For this review, take the finished solid that the model builds, in its own axes (mm). Coordinates: 2 decimals unless noted, no trailing zeros. Order: outer loops, then holes, each group sorted by start corner. A loop starts at its lowest first (then second) coordinate and runs counter-clockwise, first axis right, second up. Notation, with made-up numbers: (83.25, 11.25) -> (142.25, 11.25) arc R14 cw to (142.25, 15.25) -> close; hole circle Ø7 at (7.5, -12.75). An arc over 180 degrees is marked (long way). Return JSON: item names as keys, results as strings. Group by question number.
Item 1: Take a section at A-A (x = -3.5). Write out the cut boundary in (y, z), then the cut area to 3 significant figures.
Item 2: Take a section at C-C (y = -8.5). Write out the cut boundary in (x, z).
Item 3: Insertion check: pin 1 (4 mm diameter, centred on x = 14, y = -42, fed in from +Z); pin 2 (8 mm diameter, centred on x = -20.5, z = 17.5, fed in from +Y). Each pin has a flat end and moves straight along its axis. Give the tip position at first contact, or say it passes through.
Item 4: For line 1 along Z through (x, y) = (12, -12); line 2 along Y through (x, z) = (23, 8); line 3 along Y through (x, z) = (26, 11), list the stretches that pass through material, from the lowest coordinate up.
Item 5: Take a section at B-B (z = 20). Write out the cut boundary in (x, y), then the cut area to 3 significant figures.
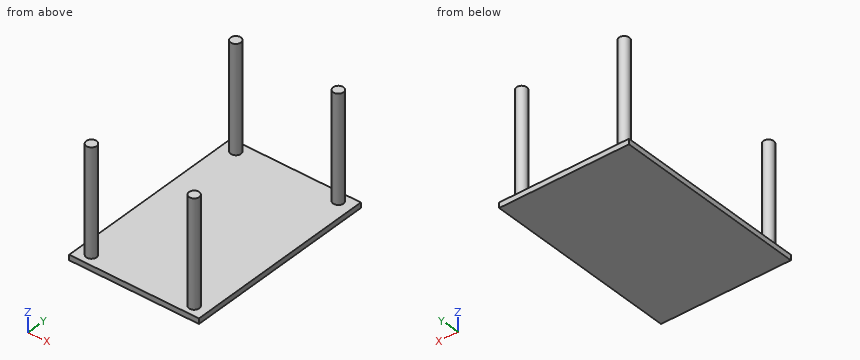
```python
from build123d import *

# Parameters (mm, degrees)
F0_W      = 61.878236
F0_H      = 93.249064
F1_DEPTH  = 2.54
F2_R      = 3.356363
F3_DEPTH  = 34.29
F4_R      = 2.475799
F5_DEPTH  = 50.8
F6_R      = 2.475799
F7_DEPTH  = 50.8
F8_R      = 2.475798
F9_DEPTH  = 50.8
F10_R     = 2.459012
F11_DEPTH = 50.8


with BuildPart() as f1:
    # F0 (on Top) → F1 (new body)
    with BuildSketch(Plane.XY):
        with Locations((-1e-06, -5.90002)):
            Rectangle(F0_W, F0_H)
    extrude(amount=F1_DEPTH)

    # F2 (on face) → F3 (cut)
    with BuildSketch(Plane(origin=(0, 0, 0), x_dir=(1, 0, 0), z_dir=(0, 0, -1))):
        with Locations((-24.319587, 47.631852)):
            Circle(F2_R)
    extrude(amount=F3_DEPTH, mode=Mode.SUBTRACT)

    # F4 (on face) → F5 (join)
    with BuildSketch(Plane.XY.offset(2.54)):
        with Locations((-24.607392, 35.831816)):
            Circle(F4_R)
    extrude(amount=F5_DEPTH)

    # F6 (on face) → F7 (join)
    with BuildSketch(Plane.XY.offset(2.54)):
        with Locations((24.031781, 36.119621)):
            Circle(F6_R)
    extrude(amount=F7_DEPTH)

    # F8 (on face) → F9 (join)
    with BuildSketch(Plane.XY.offset(2.54)):
        with Locations((-24.607392, -47.344048)):
            Circle(F8_R)
    extrude(amount=F9_DEPTH)

    # F10 (on face) → F11 (join)
    with BuildSketch(Plane.XY.offset(2.54)):
        with Locations((24.607392, -47.631852)):
            Circle(F10_R)
    extrude(amount=F11_DEPTH)


solid = f1.part
```
Findings below:
{
 "1": {"outline": "(-52.52, 0) -> (40.72, 0) -> (40.72, 2.54) -> (-52.52, 2.54) -> close", "area": "237 mm2"},
 "2": {"outline": "(-30.94, 0) -> (30.94, 0) -> (30.94, 2.54) -> (-30.94, 2.54) -> close"},
 "3": {"pin 1": "stops at z = 2.54", "pin 2": "stops at y = 38.31"},
 "4": {"line 1": "z = 0 to 2.54", "line 2": "y = -49.49 to -45.77, 33.87 to 38.37", "line 3": "y = -49.66 to -45.61, 34.62 to 37.62"},
 "5": {"outline": "circle Ø4.95 at (-24.61, -47.34); circle Ø4.95 at (-24.61, 35.83); circle Ø4.95 at (24.03, 36.12); circle Ø4.92 at (24.61, -47.63)", "area": "76.8 mm2"}
}
